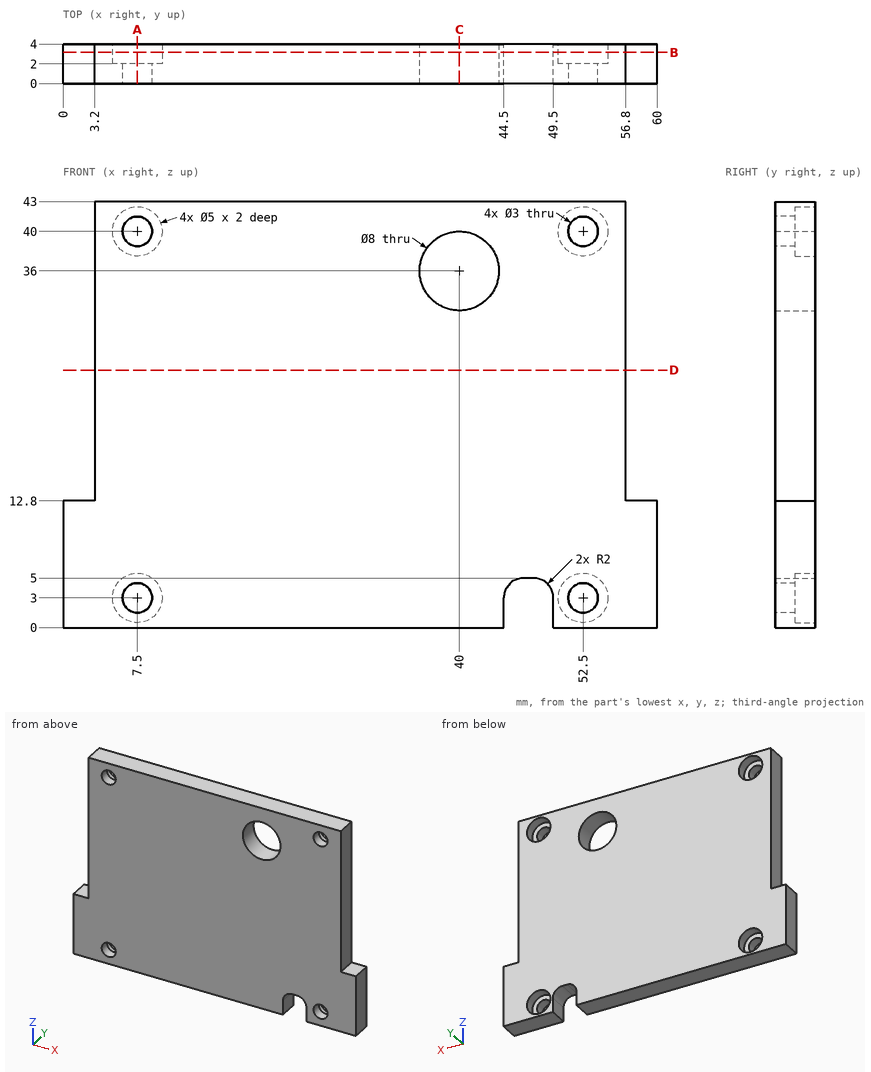
Here's the drawing with two shaded views (mm, measured from the low corner). I have some questions. Give positions to 0.01 mm unless a question says otherwise; leave off trailing zeros. Write each loop counter-clockwise with the first axis right and the second up, starting at its lowest first coordinate (ties: lowest second). Pieces come first, ordered by that corner, then holes. Notation, with made-up numbers: (15, 69) -> (54, 69) arc R13 ccw to (54, 74) -> close; hole circle Ø6 at (8.5, 36.25). An arc over 180 degrees is marked (long way). Answer as a JSON object with one key per item and string values. Group by question number.
Item 1: Suppose I cut it at A-A (x = 7.5). Please give me the cut outline in (y, z), plus the area to 3 significant figures.
Item 2: Suppose I cut it at D-D (z = 26). Please give me the cut outline in (x, y), plus the area to 3 significant figures.
Item 3: Suppose I cut it at B-B (y = 3.15). Please give me the cut outline in (x, z).
Item 4: I'm going to push flat-ended pins straight in: P1, Ø5, axis at x = 52.5, z = 40, coming from the -Y side; P2, Ø4, axis at x = 7.5, z = 40, coming from the +Y side; P3, Ø1.5, axis at y = 1, z = 35.5, coming from the +X side; P4, Ø2.5, axis at x = 7.5, z = 3, coming from the -Y side. Where does each tip first touch, or does it pass through?
Item 5: Suppose I cut it at C-C (x = 40). Please give me the cut outline in (y, z).
Item 6: Please list where these lines run through material, in increasing order: line 1 (X direction, y = 1.3, z = 3); line 2 (Z direction, x = 52.5, y = 0.9); line 3 (X direction, y = 2.65, z = 3). Write a range as [from, to].
Findings:
{
 "1": {"outline": "(0, 0) -> (4, 0) -> (4, 0.5) -> (2, 0.5) -> (2, 1.5) -> (0, 1.5) -> close; (0, 4.5) -> (2, 4.5) -> (2, 5.5) -> (4, 5.5) -> (4, 37.5) -> (2, 37.5) -> (2, 38.5) -> (0, 38.5) -> close; (0, 41.5) -> (2, 41.5) -> (2, 42.5) -> (4, 42.5) -> (4, 43) -> (0, 43) -> close", "area": "140 mm²"},
 "2": {"outline": "(3.2, 0) -> (56.8, 0) -> (56.8, 4) -> (3.2, 4) -> close", "area": "214 mm²"},
 "3": {"outline": "(0, 0) -> (44.5, 0) -> (44.5, 3) arc R2 cw to (46.5, 5) -> (47.5, 5) arc R2 cw to (49.5, 3) -> (49.5, 0) -> (60, 0) -> (60, 12.8) -> (56.8, 12.8) -> (56.8, 43) -> (3.2, 43) -> (3.2, 12.8) -> (0, 12.8) -> close; hole circle Ø5 at (7.5, 3); hole circle Ø5 at (7.5, 40); hole circle Ø8 at (40, 36); hole circle Ø5 at (52.5, 3); hole circle Ø5 at (52.5, 40)"},
 "4": {"P1": "stops at y = 0", "P2": "stops at y = 2", "P3": "stops at x = 56.8", "P4": "passes through"},
 "5": {"outline": "(0, 0) -> (4, 0) -> (4, 32) -> (0, 32) -> close; (0, 40) -> (4, 40) -> (4, 43) -> (0, 43) -> close"},
 "6": {"line 1": "x = [0, 6], [9, 44.5], [49.5, 51], [54, 60]", "line 2": "z = [0, 1.5], [4.5, 38.5], [41.5, 43]", "line 3": "x = [0, 5], [10, 44.5], [49.5, 50], [55, 60]"}
}
